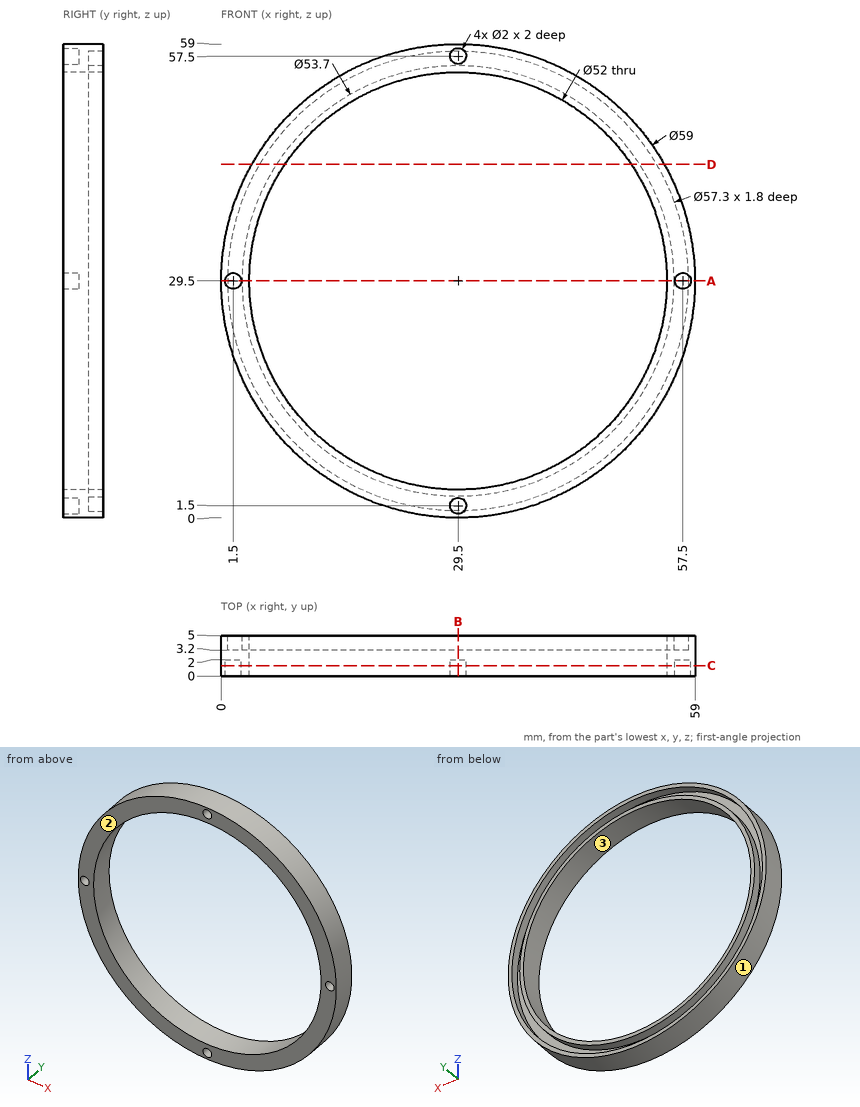
Answer from the drawing. Dimensions are ordinates in mm from the lowest x, y and z of the part. Give positions to 0.01 mm unless a question says otherwise; leave off trailing zeros. Loops run counter-clockwise (first coordinate to the right, second up) from the corner with the lowest first, then second, coordinate; pieces in that order, holes last. Notation, with made-up numbers: (53.5, 40) - (63.5, 40) arc R21 ccw to (63.5, 67) - close; hole circle Ø9 at (-9.5, 72). An arc over 180 degrees is marked (long way). Answer as a JSON object with one key per item and string values.
1. A cutting plane is placed at B-B (x = 29.5). Write down the section's boundary in (y, z), then the cut area to 3 significant figures.
Determined:
{"outline": "(0, 0) - (5, 0) - (5, 0.85) - (3.2, 0.85) - (3.2, 2.65) - (5, 2.65) - (5, 3.5) - (0, 3.5) - (0, 2.5) - (2, 2.5) - (2, 0.5) - (0, 0.5) - close; (0, 55.5) - (5, 55.5) - (5, 56.35) - (3.2, 56.35) - (3.2, 58.15) - (5, 58.15) - (5, 59) - (0, 59) - (0, 58.5) - (2, 58.5) - (2, 56.5) - (0, 56.5) - close", "area": "20.5 mm²"}
2. For a pull along X with two mould halves and no side action, classify the marked faces 1, 2 and 3 as pulls with the +X half, pulls with the -X half, needs draft (parallel to the pull), parting line crosses it, or undercut.
Determined:
{"face 1": "parting line crosses it", "face 2": "needs draft", "face 3": "undercut"}
3. Flat-ended cylindrical pins translate along their axes: pin 1 Ø1.5 at (y, z) = (1.5, 39.5) entering from -X; pin 2 Ø0.6 at (x, z) = (29.5, 58) entering from -Y; pin 3 Ø1.2 at (x, z) = (57.5, 29.5) entering from +Y; pin 4 Ø10 at (x, z) = (24, 13) entering from +Y. Find the tip coordinate at first contact, or state that the pin passes through.
Determined:
{"pin 1": "x = 1.49", "pin 2": "y = 2", "pin 3": "y = 3.2", "pin 4": "through"}
4. A cutting plane is placed at A-A (z = 29.5). Write down the section's boundary in (x, y), then the cut area to 3 significant figures.
Determined:
{"outline": "(0, 0) - (0.5, 0) - (0.5, 2) - (2.5, 2) - (2.5, 0) - (3.5, 0) - (3.5, 5) - (2.65, 5) - (2.65, 3.2) - (0.85, 3.2) - (0.85, 5) - (0, 5) - close; (55.5, 0) - (56.5, 0) - (56.5, 2) - (58.5, 2) - (58.5, 0) - (59, 0) - (59, 5) - (58.15, 5) - (58.15, 3.2) - (56.35, 3.2) - (56.35, 5) - (55.5, 5) - close", "area": "20.5 mm²"}
5. Find the intervals of material crossed by L1, parallel to Z at x = 29.5, y = 0.75; L2, parallel to X at y = 3.9, z = 52.5; L3, parallel to Z at x = 23.5, y = 2.75, in increasing order. Write a range as [from, to].
Determined:
{"L1": "[0, 0.5], [2.5, 3.5], [55.5, 56.5], [58.5, 59]", "L2": "[11.03, 12.42], [15.65, 17.38], [41.62, 43.35], [46.58, 47.97]", "L3": "[0.62, 4.2], [54.8, 58.38]"}
6. A cutting plane is placed at D-D (z = 44). Write down the section's boundary in (x, y).
Determined:
{"outline": "(3.81, 0) - (7.92, 0) - (7.92, 5) - (6.9, 5) - (6.9, 3.2) - (4.79, 3.2) - (4.79, 5) - (3.81, 5) - close; (51.08, 0) - (55.19, 0) - (55.19, 5) - (54.21, 5) - (54.21, 3.2) - (52.1, 3.2) - (52.1, 5) - (51.08, 5) - close"}
7. A cutting plane is placed at C-C (y = 1.3). Write down the section's boundary in (x, z).
Determined:
{"outline": "circle Ø59 at (29.5, 29.5); hole circle Ø2 at (1.5, 29.5); hole circle Ø52 at (29.5, 29.5); hole circle Ø2 at (29.5, 1.5); hole circle Ø2 at (29.5, 57.5); hole circle Ø2 at (57.5, 29.5)"}
